Autodesk Inventor part; units mm, degrees
ref_plane "WorkPlane1" through (0, 0, 0) normal (0, 0, 1) x (1, 0, 0)
ref_plane "MSC_PF1" through (0, 0, 0) normal (1, 0, 0) x (0, 1, 0)
ref_plane "MSC_PT1" through (0, 0, 0) normal (0, 0, -1) x (-1, 0, 0)
ref_plane "WorkPlane1" through (0, 0, 0) normal (0, 0, 1) x (1, 0, 0)
sketch "Sketch1" plane through (0, 0, 0) normal (0, 0, 1) x (1, 0, 0)
  point P0 (0, 0)
sketch "Sketch2" plane through (0, 0, 0) normal (0, 0, 1) x (1, 0, 0)
  line L0 (-8, 4.6189) -> (-8, -4.6189)
  line L1 (0, 9.2375) -> (-8, 4.6189)
  line L2 (8, 4.6189) -> (0, 9.2375)
  line L3 (8, -4.6189) -> (8, 4.6189)
  line L4 (0, -9.2375) -> (8, -4.6189)
  line L5 (-8, -4.6189) -> (0, -9.2375)
  circle A0 centre (0, 0) radius 8 construction
  dimension "d1" = 16
  dimension "d29" = 0
  dimension "d30" = 0
extrude "Extrusion1" add sketch "Sketch2" along normal blind 6.4
sketch "Sketch3" plane through (0, 0, 0) normal (1, 0, 0) x (0, 1, 0)
  line L0 (8, 6.4) -> (9.3375, 6.4)
  line L1 (9.3375, 5.6278) -> (8, 6.4)
  line L2 (9.3375, 6.4) -> (9.3375, 5.6278)
  line L3 (0, -1.28) -> (0, 7.68)
  line L4 (9.2375, 0) -> (9.2375, 6.4)
  dimension "d25" = 0.1
  dimension "d26" = 0
  dimension "d27" = 60
  dimension "d28" = 8
revolve "Revolution1" cut sketch "Sketch3" angle 360 about axis through (0, 0, -10) along (0, 0, 1)
sketch "Sketch4" plane through (0, 0, 0) normal (1, 0, 0) x (0, 1, 0)
  line L0 (0, -45) -> (0, 0)
  line L1 (-5, -45) -> (0, -45)
  line L2 (-5, 0) -> (-5, -45)
  line L3 (0, 0) -> (-5, 0)
  line L4 (0, -45) -> (0, 0)
  line L5 (-6, 0) -> (1, 0)
  line L6 (0, -54) -> (0, 9)
  dimension "d18" = 5
  dimension "d20" = 45
  dimension "d33" = 0
  dimension "d34" = 0
revolve "Revolution2" add sketch "Sketch4" angle 360 about axis through (0, 0, -45) along (0, 0, -1)
chamfer "Chamfer1" distance 0.75 angle 45 1 edges at (0, 5, -45)
fillet "Fillet1" radius 0.4 1 edges at (0, 5, 0)
thread "Thread1"
ref_plane "MSC_PF1" through (0, 0, 0) normal (1, 0, 0) x (0, 1, 0)
ref_plane "MSC_PT1" through (0, 0, 0) normal (0, 0, -1) x (-1, 0, 0)
equation "\"d22\" = 0.5 * PTC"
equation "\"d23\" = 0.5 * PTC"
equation "\"d24\" = r"
equation "\"d1\" = ParS"
equation "\"d6\" = ParK"
equation "\"d28\" = 0.5 * ParS"
equation "\"d18\" = 0.5 * NND"
equation "\"d20\" = NLG"
equation "\"NLG\" = 45"
equation "\"PTC\" = 1.5"
equation "\"ParK\" = 6.4"
equation "\"ParS\" = 16"
equation "\"msp_es\" = 0.577367 * ParS"
equation "\"r\" = 0.4"
properties part number "ISO 4016 - M10 x 45" material "Steel"
Geometry check sheet. Reference: the model listing, model coordinates, mm. A direction names the side the tool comes from. Coordinates: 2 decimals unless noted, no trailing zeros. Loops run counter-clockwise (first coordinate to the right, second up) from the corner with the lowest first, then second, coordinate; pieces in that order, holes last. Notation, with made-up numbers: (-26.5, 86.5) -> (2.5, 86.5) arc R20 ccw to (2.5, 107.5) -> close; hole circle Ø1 at (-37.5, -23.75). An arc over 180 degrees is marked (long way). Put each result on its own line as item: value.
1) Thickness scan on line 1 (Y direction, x = 0, z = -20.5); line 2 (Z direction, x = 3.5, y = -6.25); line 3 (X direction, y = -3, z = -20). Record the ranges inside material, lowest first.
Result set:
line 1: y = -5 to 5
line 2: z = 0 to 6.4
line 3: x = -4 to 4
2) Cross-section at A-A on z = -11.5. Record the boundary of the cut face in (x, y), plus the area to 3 significant figures.
Result set:
outline: circle Ø10 at (0, 0)
area: 78.5 mm^2
3) Tool access check on faces 1 (the conical face through (-7.179, -4.168, 6.226)), 2 (the flat face through (-4, -4, 0)). Record the directions out of +Z, -Z, +X, -X, +Y, -Y that give a thin tool (end or side, any length) a straight path to the whole face; none if there is none.
Result set:
face 1: +Z, -X, -Y
face 2: -Z
4) Gauge pin test, flat ends, axial feed: pin 1 Ø2 at (x, z) = (-5.5, -9) entering from -Y; pin 2 Ø1.5 at (x, y) = (-5.5, 1.5) entering from -Z; pin 3 Ø8 at (x, z) = (-2.5, -5.5) entering from +Y. Record the tip position at first contact, or that the pin passes through.
Result set:
pin 1: stops at y = -2.18
pin 2: stops at z = -44.3
pin 3: stops at y = 5
